from build123d import *

# Parameters (mm, degrees)
SKETCH1_R           = 4
SKETCH1_R_2         = 2
SKETCH1_R_3         = 1.25
BOSS_EXTRUDE1_DEPTH = 5


with BuildPart() as part:
    # Sketch1 → Boss-Extrude1 (new body)
    with BuildSketch(Plane.XY):
        with BuildLine():
            Line((-32.5, 60), (-52.5, 60))
            Line((-52.5, 60), (-52.5, 33.860836522))
            ThreePointArc((-52.5, 33.860836522), (-83.9125, 0), (-52.5, -33.860836522))
            Line((-52.5, -33.860836522), (-52.5, -60))
            Line((-52.5, -60), (52.5, -60))
            Line((52.5, -60), (52.5, -33.860836522))
            ThreePointArc((52.5, -33.860836522), (83.9125, 0), (52.5, 33.860836522))
            Line((52.5, 33.860836522), (52.5, 60))
            Line((52.5, 60), (32.5, 60))
            Line((32.5, 60), (32.5, 45))
            Line((32.5, 45), (-32.5, 45))
            Line((-32.5, 45), (-32.5, 60))
        make_face()
        with Locations((-49.95625, 0)):
            Circle(SKETCH1_R, mode=Mode.SUBTRACT)
        with Locations((-27, -39)):
            Circle(SKETCH1_R_2, mode=Mode.SUBTRACT)
        with Locations((27, -39)):
            Circle(SKETCH1_R_2, mode=Mode.SUBTRACT)
        with Locations((-27, 33)):
            Circle(SKETCH1_R_2, mode=Mode.SUBTRACT)
        with Locations((-47.5, 45)):
            Circle(SKETCH1_R_2, mode=Mode.SUBTRACT)
        with Locations((27, 33)):
            Circle(SKETCH1_R_2, mode=Mode.SUBTRACT)
        with Locations((47.5, 45)):
            Circle(SKETCH1_R_2, mode=Mode.SUBTRACT)
        with Locations((-41.95625, 0)):
            Circle(SKETCH1_R_3, mode=Mode.SUBTRACT)
        with Locations((-49.95625, 9.5)):
            Circle(SKETCH1_R_3, mode=Mode.SUBTRACT)
        with Locations((-49.95625, -9.5)):
            Circle(SKETCH1_R_3, mode=Mode.SUBTRACT)
        with Locations((-57.95625, 0)):
            Circle(SKETCH1_R_3, mode=Mode.SUBTRACT)
        with Locations((49.95625, 9.5)):
            Circle(SKETCH1_R_3, mode=Mode.SUBTRACT)
        with Locations((49.95625, -9.5)):
            Circle(SKETCH1_R_3, mode=Mode.SUBTRACT)
        with Locations((41.95625, 0)):
            Circle(SKETCH1_R_3, mode=Mode.SUBTRACT)
        with Locations((57.95625, 0)):
            Circle(SKETCH1_R_3, mode=Mode.SUBTRACT)
    extrude(amount=BOSS_EXTRUDE1_DEPTH)


solid = part.part
Could you check a few things on this model? Use its own coordinates, in mm. A direction names the side the tool comes from. Round coordinates to 2 decimals unless told otherwise and drop trailing zeros. Loops run counter-clockwise (first coordinate to the right, second up) from the corner with the lowest first, then second, coordinate; pieces in that order, holes last. Notation, with made-up numbers: (-30, 24) -> (25, 24) arc R21 cw to (25, 36) -> close; hole circle Ø7 at (29.5, -36.75). An arc over 180 degrees is marked (long way). Use CSV: the item, a comma, the result in double quotes.
(1) Suppose I cut it at D-D on z = 3.4. Give the number of separate pieces and of enclosed holes in the cut face, plus the area to 3 significant figures.
Return value:
separate pieces,"1"
enclosed holes,"15"
area,"14,700 mm²"
(2) For faces 1 (the flat face through (-32.5, 52, 2)), 2 (the cylindrical face through (-47.934, 43.048, 2.465)), 3 (the flat face through (52.5, -47, 2)), 4 (the flat face through (-52.5, 47, 2)), 5 (the flat face through (52.5, 47, 2)), which set-ups out of +Z, -Z, +X, -X, +Y, -Y let a thin tool reach every point of the face, with its end or its side?
Return value:
face 1,"+Z, -Z, +Y"
face 2,"+Z, -Z"
face 3,"+Z, -Z, +X, -Y"
face 4,"+Z, -Z, -X, +Y"
face 5,"+Z, -Z, +X, +Y"
(3) Suppose I cut it at C-C on y = -39. Write out the boundary of the cut face in (x, z), plus the area to 3 significant figures.
Return value:
outline,"(-52.5, 0) -> (-29, 0) -> (-29, 5) -> (-52.5, 5) -> close; (-25, 0) -> (25, 0) -> (25, 5) -> (-25, 5) -> close; (29, 0) -> (52.5, 0) -> (52.5, 5) -> (29, 5) -> close"
area,"485 mm²"
(4) Suppose I cut it at B-B on x = 27. Write out the boundary of the cut face in (y, z), plus the area to 3 significant figures.
Return value:
outline,"(-60, 0) -> (-41, 0) -> (-41, 5) -> (-60, 5) -> close; (-37, 0) -> (31, 0) -> (31, 5) -> (-37, 5) -> close; (35, 0) -> (45, 0) -> (45, 5) -> (35, 5) -> close"
area,"485 mm²"
(5) If I drill on probe 1 along Y at (x, z) = (-21.5, 1.75); probe 2 along X at (y, z) = (-53.5, 2.75); probe 3 along Y at (x, z) = (-57.5, 3.45), over which ranges is the centre line in solid material (lowest first)? Write a range as [from, to].
Return value:
probe 1,"y = [-60, 45]"
probe 2,"x = [-52.5, 52.5]"
probe 3,"y = [-33.11, -1.16], [1.16, 33.11]"
(6) Will these pins go through, and if not, where does the flat tip stop? pin 1 Ø3 at (x, y) = (49.96, -9.5) entering from +Z; pin 2 Ø2 at (x, y) = (49.96, 9.5) entering from -Z; pin 3 Ø2.5 at (x, z) = (12, 1.5) entering from +Y; pin 4 Ø2 at (y, z) = (36, 3.5) entering from +X.
Return value:
pin 1,"stops at z = 5"
pin 2,"passes through"
pin 3,"stops at y = 45"
pin 4,"stops at x = 52.5"
(7) If we mould it in two halves opening along X, with no side actions, what happens to faces 6 (the flat face through (-42, 60, 2)), 7 (the flat face through (32.5, 53, 2)), 8 (the cylindrical face through (83.905, -0.711, 2.465)), 9 (the flat face through (-52.5, -47, 2))? For each: +X half, -X half, draft (parallel to the pull), parting line (faces both ways), or undercut.
Return value:
face 6,"draft"
face 7,"undercut"
face 8,"+X half"
face 9,"-X half"
(8) Suppose I cut it at A-A on y = 52. Write out the boundary of the cut face in (x, z), plus the area to 3 significant figures.
Return value:
outline,"(-52.5, 0) -> (-32.5, 0) -> (-32.5, 5) -> (-52.5, 5) -> close; (32.5, 0) -> (52.5, 0) -> (52.5, 5) -> (32.5, 5) -> close"
area,"200 mm²"
